The model under review builds one solid part; all positions refer to its coordinate system, in mm. A direction names the side the tool comes from. Coordinates: 2 decimals unless noted, no trailing zeros. Loops run counter-clockwise (first coordinate to the right, second up) from the corner with the lowest first, then second, coordinate; pieces in that order, holes last. Notation, with made-up numbers: M 39.25,-20 L 47.25,-20 A23 ccw 47.25,5 Z; hole C 2,36.25 d4. An arc over 180 degrees is marked long. Use one line per item in the form item = value.
Autodesk Inventor part; units mm, degrees
ref_plane "YZ Plane" through (0, 0, 0) normal (1, 0, 0) x (0, 1, 0)
ref_plane "XZ Plane" through (0, 0, 0) normal (0, 1, 0) x (-1, 0, 0)
ref_plane "XY Plane" through (0, 0, 0) normal (0, 0, 1) x (1, 0, 0)
sketch "草圖2" plane through (0, 0, 0) normal (0, 1, 0) x (-1, 0, 0)
  line L0 (-2.8868, 0) -> (-1.4434, 2.5)
  line L1 (-1.4434, 2.5) -> (1.4434, 2.5)
  line L2 (1.4434, 2.5) -> (2.8868, 0)
  line L3 (2.8868, 0) -> (1.4434, -2.5)
  line L4 (1.4434, -2.5) -> (-1.4434, -2.5)
  line L5 (-1.4434, -2.5) -> (-2.8868, 0)
  point P0 (0, 0)
  point P1 (0, 0)
  dimension "d2" = 5
extrude "擠出1" add sketch "草圖2" along normal blind 20
sketch "草圖3" plane through (0, 0, 0) normal (0, 0, 1) x (1, 0, 0)
  line L0 (1.4434, 20) -> (-1.4434, 20)
  line L1 (0, 20) -> (1.5, 20)
  line L2 (1.5, 20) -> (1.5, 26)
  line L3 (1.5, 26) -> (0, 26)
  line L4 (0, 26) -> (0, 20)
  line L5 (0, 17.268) -> (0, -3.3114)
  line L6 (0, 0) -> (1.5, 0)
  line L7 (1.5, 0) -> (1.5, -6)
  line L8 (1.5, -6) -> (0, -6)
  line L9 (0, -6) -> (0, 0)
  point P0 (0.75, 26)
  dimension "d5" = 3
  dimension "d6" = 6
  dimension "d8" = 6
revolve "迴轉1" add sketch "草圖3" angle 360 about axis through (0, 17.268, 0) along (0, -1, 0)
properties part number "copper_pillar_M3_L25"
1. Insertion check: P1, Ø1.5, axis at y = 5, z = 2, coming from the -X side; P2, Ø1.5, axis at y = 8, z = -0.5, coming from the +X side. Each pin has a flat end and moves straight along its axis. Give the tip position at first contact, or say it passes through.
Response values:
P1 = -2.17
P2 = 2.89
2. Wall thickness on line 1 along Y through (x, z) = (-2.05, 0.8); line 2 along Z through (x, y) = (1.2, -3); line 3 along X through (y, z) = (17.5, -2.15): over which ranges is each line inside the solid? List them lowest first. Write a range as from..to.
Response values:
line_1 = 0..20
line_2 = -0.9..0.9
line_3 = -1.65..1.65
3. Add section B-B (y = 1). State the section outline as (x, z) points, then the cut area to 3 significant figures.
Response values:
outline = M -2.89,0 L -1.44,-2.5 L 1.44,-2.5 L 2.89,0 L 1.44,2.5 L -1.44,2.5 Z
area = 21.7 mm^2
4. Add section A-A (x = 0). State the section outline as (y, z) points, then the cut area to 3 significant figures.
Response values:
outline = M -6,-1.5 L 0,-1.5 L 0,-2.5 L 20,-2.5 L 20,-1.5 L 26,-1.5 L 26,1.5 L 20,1.5 L 20,2.5 L 0,2.5 L 0,1.5 L -6,1.5 Z
area = 136 mm^2
5. Add section D-D (z = -2.15). State the section outline as (x, y) points, then the cut area to 3 significant figures.
Response values:
outline = M -1.65,0 L 1.65,0 L 1.65,20 L -1.65,20 Z
area = 65.8 mm^2
6. Machinability: for faces 1 (the face through (2.155, 9.86, -1.267)), 2 (the face through (-1.5, 23.04, -0.07)), 3 (the face through (-1.5, -3.04, 0.07)), which of the approach directions +Z, -Z, +X, -X, +Y, -Y give a long, thin tool a straight path to every point of the face, cutting with its end or side? Answer none if there is none.
Response values:
face_1 = -Z, +X, +Y, -Y
face_2 = +Y
face_3 = -Y
7. Add section C-C (z = 0.75). State the section outline as (x, y) points, then the cut area to 3 significant figures.
Response values:
outline = M -2.45,0 L -1.3,0 L -1.3,-6 L 1.3,-6 L 1.3,0 L 2.45,0 L 2.45,20 L 1.3,20 L 1.3,26 L -1.3,26 L -1.3,20 L -2.45,20 Z
area = 129 mm^2
